Build history of the part. All positions in model axes, mm. Round coordinates to 2 decimals unless told otherwise and drop trailing zeros. Write each loop counter-clockwise with the first axis right and the second up, starting at its lowest first coordinate (ties: lowest second). Pieces come first, ordered by that corner, then holes. Notation, with made-up numbers: (73, 17.25) -> (109, 17.25) arc R15 ccw to (109, 21.25) -> close; hole circle Ø6 at (53, 7.25). An arc over 180 degrees is marked (long way). Answer as CSV lines item,"result".
Autodesk Inventor part; units mm, degrees
ref_plane "YZ Plane" through (0, 0, 0) normal (1, 0, 0) x (0, 1, 0)
ref_plane "XZ Plane" through (0, 0, 0) normal (0, 1, 0) x (-1, 0, 0)
ref_plane "XY Plane" through (0, 0, 0) normal (0, 0, 1) x (1, 0, 0)
sketch "Esquisse1" plane through (0, 0, 0) normal (0, 0, 1) x (1, 0, 0)
  line L0 (-63, 0) -> (63, 0) construction
  line L1 (-60, -3) -> (60, -3)
  line L2 (60, 3) -> (-60, 3)
  arc A0 (-60, 3) -> (-60, -3) centre (-60, 0) ccw
  arc A1 (60, -3) -> (60, 3) centre (60, 0) ccw
  line L3 (0, -4.2) -> (0, 4.2)
  circle A2 centre (-60, 0) radius 1.5
  circle A3 centre (60, 0) radius 1.5
  circle A4 centre (5.35, 0) radius 1.5
  point P0 (0, 0)
  point P1 (0, 0)
  dimension "d0" = 120
  dimension "d1" = 6
  dimension "d2" = 3
  dimension "d4" = 3
  dimension "d7" = 3
  dimension "d9" = 54.65
extrude "Extrusion1" add sketch "Esquisse1" along normal mid plane 3
properties part number "barre_direction"
1. Drop a flat-ended pin along its axis: pin 1 Ø3.5 at (x, y) = (5.35, 0) entering from +Z. Give the stop position or say it passes through.
Results found:
pin 1,"stops at z = 1.5"
2. Cut at A-A, the plane x = 5.35. Write the cut outline in (y, z), then the cut area to 3 significant figures.
Results found:
outline,"(-3, -1.5) -> (-1.5, -1.5) -> (-1.5, 1.5) -> (-3, 1.5) -> close; (1.5, -1.5) -> (3, -1.5) -> (3, 1.5) -> (1.5, 1.5) -> close"
area,"9.00 mm2"
3. Mould opens along Y. For faces 1 (the cylindrical face through (63, 0, 0)), 2 (the cylindrical face through (-58.57, -0.45, -0.02)), 3 (the cylindrical face through (61.43, -0.45, -0.02)), 4 (the flat face through (1, 3, 0)) say: +Y half, -Y half, draft (parallel to the pull), parting line (faces both ways), or undercut.
Results found:
face 1,"parting line"
face 2,"undercut"
face 3,"undercut"
face 4,"+Y half"
4. Cut at B-B, the plane z = 0.8. Write the cut outline in (x, y), then the cut area to 3 significant figures.
Results found:
outline,"(-60, -3) -> (60, -3) arc R3 ccw to (60, 3) -> (-60, 3) arc R3 ccw to start; hole circle Ø3 at (-60, 0); hole circle Ø3 at (5.35, 0); hole circle Ø3 at (60, 0)"
area,"727 mm2"
5. Probe line 1 along Y through (x, z) = (-60, 0.75); line 2 along X through (y, z) = (-1, -1.25); line 3 along X through (y, z) = (-0.4, -0.7). List the from-to ranges inside material, lowest first.
Results found:
line 1,"y = -3 to -1.5, 1.5 to 3"
line 2,"x = -62.83 to -61.12, -58.88 to 4.23, 6.47 to 58.88, 61.12 to 62.83"
line 3,"x = -62.97 to -61.45, -58.55 to 3.9, 6.8 to 58.55, 61.45 to 62.97"
6. Cut at C-C, the plane y = 0. Write the cut outline in (x, z).
Results found:
outline,"(-63, -1.5) -> (-61.5, -1.5) -> (-61.5, 1.5) -> (-63, 1.5) -> close; (-58.5, -1.5) -> (3.85, -1.5) -> (3.85, 1.5) -> (-58.5, 1.5) -> close; (6.85, -1.5) -> (58.5, -1.5) -> (58.5, 1.5) -> (6.85, 1.5) -> close; (61.5, -1.5) -> (63, -1.5) -> (63, 1.5) -> (61.5, 1.5) -> close"
